```python
from build123d import *

# Parameters (mm, degrees)
F0_W     = 26.6334357138
F0_H     = 19.05
F1_DEPTH = 25.4
F2_DEPTH = 63.5
F3_DEPTH = 7.9375
F4_R     = 5.08


with BuildPart() as f1:
    # F0 (on Front) → F1 (new body, symmetric)
    with BuildSketch(Plane.XZ):
        with BuildLine():
            Line((22.225, 9.525), (41.275, 9.525))
            Line((41.275, 9.525), (41.275, 27.0002))
            ThreePointArc((41.275, 27.0002), (45.9246798487, 38.2255201513), (57.15, 42.8752))
            Line((57.15, 42.8752), (60.325, 42.8752))
            Line((60.325, 42.8752), (60.325, 61.9252))
            Line((60.325, 61.9252), (57.15, 61.9252))
            add(Edge.make_bspline(
                [(56.6413277741, 61.9214954738), (56.8116800634, 61.9231681109), (56.9812416063, 61.9244029276), (57.15, 61.9252)],
                knots=[110.9405929151, 110.9405929151, 110.9405929151, 110.9405929151, 111.5045361635, 111.5045361635, 111.5045361635, 111.5045361635], degree=3))
            ThreePointArc((56.6413277741, 61.9214954738), (32.2751029903, 51.515401891), (22.225, 27.0002))
            Line((22.225, 27.0002), (22.225, 9.525))
        make_face()
        with Locations((73.6417178569, 52.4002)):
            Rectangle(F0_W, F0_H)
    extrude(amount=F1_DEPTH, both=True)

    # F0 (on Front) → F2 (join, symmetric)
    with BuildSketch(Plane.XZ):
        Polygon((-41.275, 9.525), (-41.275, -9.525), (41.275, -9.525), (41.275, 9.525), (22.225, 9.525), align=None)
    extrude(amount=F2_DEPTH, both=True)

    # F0 (on Front) → F3 (join, symmetric)
    with BuildSketch(Plane.XZ):
        with BuildLine():
            add(Edge.make_bspline(
                [(-41.275, 9.525), (-40.9849167943, 44.3197871826), (23.1291188202, 61.5924493311), (56.6413277741, 61.9214954738)],
                knots=[0, 0, 0, 0, 110.9405929151, 110.9405929151, 110.9405929151, 110.9405929151], degree=3))
            Line((-41.275, 9.525), (22.225, 9.525))
            Line((22.225, 9.525), (22.225, 27.0002))
            ThreePointArc((22.225, 27.0002), (32.2751029903, 51.515401891), (56.6413277741, 61.9214954738))
        make_face()
    extrude(amount=F3_DEPTH, both=True)

    # F4
    f4_edges = [f1.edges().sort_by_distance(p)[0] for p in [
        (-41.275, 63.5, 0),
        (41.275, 63.5, 0),
        (41.275, -63.5, 0),
        (-41.275, -63.5, 0),
    ]]
    fillet(f4_edges, radius=F4_R)

    # F0 (on Front) → F5 (revolve)
    with BuildSketch(Plane.XZ):
        Polygon((86.9584357138, 66.675), (86.9584357138, 61.9252), (86.9584357138, 42.8752), (86.9584357138, 38.1), (111.125, 38.1), (111.125, 66.675), align=None)
    revolve(axis=Axis((86.9584357138, 0, 52.3875), (0, 0, 1)))


solid = f1.part
```
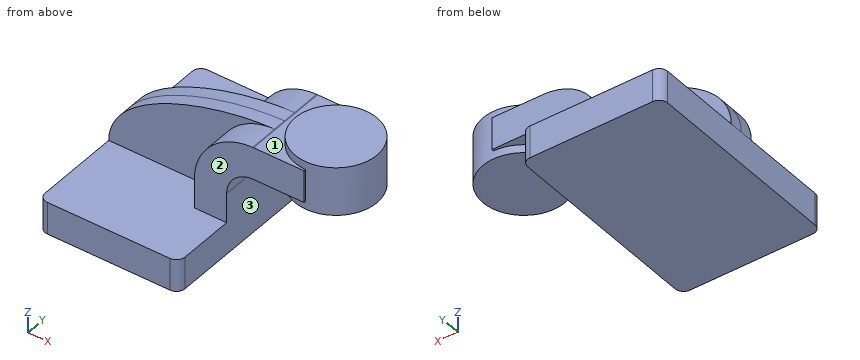
Design review of the part built by this model. Coordinates are the model's own, in mm. Face numbers are marked on the shaded views. A direction names the side the tool comes from. Give positions to 0.01 mm unless a question says otherwise; leave off trailing zeros. Write each loop counter-clockwise with the first axis right and the second up, starting at its lowest first coordinate (ties: lowest second). Pieces come first, ordered by that corner, then holes.
(1) Clearance check with flat-ended pins moving along their axes: pin 1 Ø1.4 at (y, z) = (25, 54.5) entering from +X; pin 2 Ø8 at (y, z) = (-8, 47.5) entering from -X; pin 3 Ø12 at (y, z) = (21.5, 20) entering from -X (3 decimals). State where each tip first meets the part, or that it passes through.
Checked values:
pin 1: stops at x = 86.96
pin 2: stops at x = -15.29
pin 3: stops at x = 22.225
(2) Add section B-B (y = -49). Give the boundary of the cut face in (x, z) (3 decimals), and give its area (3 significant figures).
Checked values:
outline: (-41.275, -9.525) - (41.275, -9.525) - (41.275, 9.525) - (-41.275, 9.525) - close
area: 1,570 mm2
(3) Tool access review of the marked faces 1, 2 and 3: name each direction out of +Z, -Z, +X, -X, +Y, -Y from which nothing blocks a thin tool from reaching the whole face with its end or side.
Checked values:
face 1: +Z, -X
face 2: +Z, +X, -X, -Y
face 3: -Z, +X, +Y, -Y
(4) Add section A-A (x = 66.5). Give the boundary of the cut face in (y, z) (3 decimals), and give its area (3 significant figures).
Checked values:
outline: (-25.4, 42.875) - (-12.864, 42.875) - (-12.864, 38.1) - (12.864, 38.1) - (12.864, 42.875) - (25.4, 42.875) - (25.4, 61.925) - (12.864, 61.925) - (12.864, 66.675) - (-12.864, 66.675) - (-12.864, 61.925) - (-25.4, 61.925) - close
area: 1,210 mm2
(5) Wall thickness on line 1 along Y through (x, z) = (68.5, 50); line 2 along X through (y, z) = (19.5, 6) (3 decimals); line 3 along X through (y, z) = (-17, 27.5): over which ranges is each line inside the solid? List them lowest first.
Checked values:
line 1: y = -25.4 to 25.4
line 2: x = -41.275 to 41.275
line 3: x = 22.23 to 41.28
